The listing builds one solid part. Answer for the finished solid, in the listing's coordinates (mm). A direction names the side the tool comes from. Give positions to 0.01 mm unless a question says otherwise; leave off trailing zeros. Loops run counter-clockwise (first coordinate to the right, second up) from the corner with the lowest first, then second, coordinate; pieces in that order, holes last. Notation, with made-up numbers: (-37, 35) - (12, 35) arc R32 cw to (12, 63) - close; hole circle Ø6 at (40.25, 8). An arc over 180 degrees is marked (long way). Answer in a Markdown table with one row per item. Add a question column.
```python
from build123d import *

# Parameters (mm, degrees)
EXTRUDE_1_DEPTH     = 5
SKETCH_2_R          = 2
SKETCH_2_R_2        = 5
SKETCH_2_R_3        = 12
CUT_EXTRUDE_1_DEPTH = 96.753903315
SKETCH_3_R          = 1.5
CUT_EXTRUDE_2_DEPTH = 96.753903315
CUT_EXTRUDE_4_DEPTH = 96.753903315
FILLET_1_R          = 2
FILLET_2_R          = 2
SKETCH_5_R          = 1.5
CUT_EXTRUDE_5_DEPTH = 10


with BuildPart() as part:
    # 草图1 → 凸台-拉伸1 (new body)
    with BuildSketch(Plane(origin=(0, 0, 0), x_dir=(1, 0, 0), z_dir=(0, 1, 0))):
        Polygon((20, -34.641016151), (40, 0), (20, 34.641016151), (13.095477456, 46.6), (-83.5, 46.6), (-83.5, 26.6), (-40, 26.6), (-32.32124142, 13.3), (-40, 0), (-20, -34.641016151), align=None)
    extrude(amount=EXTRUDE_1_DEPTH)

    # 草图2 → 切除-拉伸1 (cut, through all)
    with BuildSketch(Plane(origin=(0, 5, 0), x_dir=(1, 0, 0), z_dir=(0, 1, 0))):
        with Locations(Location((0, 29, 0), (0, 0, 270))):
            Circle(SKETCH_2_R)
        with Locations(Location((25.11473671, -14.5, 0), (0, 0, 270))):
            Circle(SKETCH_2_R)
        with Locations(Location((-25.11473671, -14.5, 0), (0, 0, 270))):
            Circle(SKETCH_2_R)
        with Locations(Location((0, 19.25, 0), (0, 0, 270))):
            Circle(SKETCH_2_R_2)
        with Locations(Location((0, 0, 0), (0, 0, 270))):
            Circle(SKETCH_2_R_3)
        with Locations(Location((16.670989023, -9.625, 0), (0, 0, 270))):
            Circle(SKETCH_2_R_2)
        with Locations(Location((-16.670989023, -9.625, 0), (0, 0, 270))):
            Circle(SKETCH_2_R_2)
    extrude(amount=-CUT_EXTRUDE_1_DEPTH, mode=Mode.SUBTRACT)

    # 草图3 → 切除-拉伸2 (cut, through all)
    with BuildSketch(Plane.XZ):
        with Locations(Location((-78.5, -29.6, 0), (0, 0, 270))):
            Circle(SKETCH_3_R)
        with Locations(Location((-58.5, -29.6, 0), (0, 0, 270))):
            Circle(SKETCH_3_R)
        with Locations(Location((-58.5, -43.6, 0), (0, 0, 90))):
            Circle(SKETCH_3_R)
        with Locations(Location((-78.5, -43.6, 0), (0, 0, 90))):
            Circle(SKETCH_3_R)
    extrude(amount=-CUT_EXTRUDE_2_DEPTH, mode=Mode.SUBTRACT)

    # 草图4 → 切除-拉伸4 (cut, through all)
    with BuildSketch(Plane.XZ):
        with BuildLine():
            ThreePointArc((-16.995979196, -0.369717674), (-22.006018762, 1.167018108), (-25.550949616, 5.026489386))
            Line((-25.550949616, 5.026489386), (-28.452994616, 0))
            Line((-28.452994616, 0), (-14.226497308, -24.641016151))
            Line((-14.226497308, -24.641016151), (-8.422407308, -24.641016151))
            ThreePointArc((-8.422407308, -24.641016151), (-9.992342053, -19.641280338), (-8.818174496, -14.534090909))
            ThreePointArc((-8.818174496, -14.534090909), (-14.722431864, -8.5), (-16.995979196, -0.369717674))
        make_face()
        with BuildLine():
            Line((28.452994616, 0), (25.550949616, 5.026489386))
            ThreePointArc((25.550949616, 5.026489386), (22.006018762, 1.167018108), (16.995979196, -0.369717674))
            ThreePointArc((16.995979196, -0.369717674), (14.722431864, -8.5), (8.818174496, -14.534090909))
            ThreePointArc((8.818174496, -14.534090909), (9.700044973, -16.819130296), (10, -19.25))
            ThreePointArc((10, -19.25), (9.597501578, -22.058551844), (8.422407308, -24.641016151))
            Line((8.422407308, -24.641016151), (14.226497308, -24.641016151))
            Line((14.226497308, -24.641016151), (28.452994616, 0))
        make_face()
        with BuildLine():
            Line((17.128542308, 19.614526765), (14.226497308, 24.641016151))
            Line((14.226497308, 24.641016151), (-14.226497308, 24.641016151))
            Line((-14.226497308, 24.641016151), (-17.128542308, 19.614526765))
            ThreePointArc((-17.128542308, 19.614526765), (-12.013676709, 18.47426223), (-8.1778047, 14.903808583))
            ThreePointArc((-8.1778047, 14.903808583), (0, 17), (8.1778047, 14.903808583))
            ThreePointArc((8.1778047, 14.903808583), (12.013676709, 18.47426223), (17.128542308, 19.614526765))
        make_face()
    extrude(amount=-CUT_EXTRUDE_4_DEPTH, mode=Mode.SUBTRACT)

    # 圆角1
    fillet_1_edges = [part.edges().sort_by_distance(p)[0] for p in [
        (-8.1778047, 2.5, 14.903808583),
        (-17.128542308, 2.5, 19.614526765),
        (-14.226497308, 2.5, 24.641016151),
        (14.226497308, 2.5, 24.641016151),
        (17.128542308, 2.5, 19.614526765),
        (8.1778047, 2.5, 14.903808583),
        (16.995979196, 2.5, -0.369717674),
        (25.550949616, 2.5, 5.026489386),
        (28.452994616, 2.5, 0),
        (14.226497308, 2.5, -24.641016151),
        (8.422407308, 2.5, -24.641016151),
        (8.818174496, 2.5, -14.534090909),
        (-25.550949616, 2.5, 5.026489386),
        (-16.995979196, 2.5, -0.369717674),
        (-8.818174496, 2.5, -14.534090909),
        (-8.422407308, 2.5, -24.641016151),
        (-14.226497308, 2.5, -24.641016151),
        (-28.452994616, 2.5, 0),
    ]]
    fillet(fillet_1_edges, radius=FILLET_1_R)

    # 圆角2
    fillet_2_edges = [part.edges().sort_by_distance(p)[0] for p in [
        (-20, 2.5, 34.641016151),
        (-40, 2.5, 0),
        (-32.32124142, 2.5, -13.3),
        (-40, 2.5, -26.6),
        (-83.5, 2.5, -26.6),
        (-83.5, 2.5, -46.6),
        (13.095477456, 2.5, -46.6),
        (40, 2.5, 0),
        (20, 2.5, 34.641016151),
    ]]
    fillet(fillet_2_edges, radius=FILLET_2_R)

    # 草图5 → 切除-拉伸5 (cut)
    with BuildSketch(Plane.XZ):
        with Locations(Location((-31.401807915, -29.375609946, 0), (0, 0, 270))):
            Circle(SKETCH_5_R)
        with Locations(Location((-14.716714858, -40.403196703, 0), (0, 0, 270))):
            Circle(SKETCH_5_R)
        with Locations(Location((5.152091527, -42.690232523, 0), (0, 0, 270))):
            Circle(SKETCH_5_R)
        with Locations(Location((-34.847908473, -42.690232523, 0), (0, 0, 270))):
            Circle(SKETCH_5_R)
    extrude(amount=-CUT_EXTRUDE_5_DEPTH, mode=Mode.SUBTRACT)


solid = part.part
```
(1) Given pin 1 Ø14.5 at (x, z) = (0, 0) entering from +Y; pin 2 Ø3 at (x, y) = (-22, 3.5) entering from +Z, each flat-ended and moving along its own axis, determine where each tip first touches the part or whether it passes through.
(2) A cutting plane is placed at C-C on y = 3.25. Give the number of separate pieces and of enclosed holes in the cut face, plus the area to 3 significant figures.
(3) A cutting plane is placed at A-A on z = 6.5. Determine the outline of the cut face in (x, y).
(4) Find the intervals of material crossed by line 1 along X through (y, z) = (3.6, -43.6); line 2 along Z through (x, y) = (-12.5, 1.05); line 3 along Z through (x, y) = (-24.5, 2.6), in increasing order. Write a range as [from, to].
(5) The mould has two halves that part along Z. Classify faces 3 (the face through (-34, 2, -46.6)), 4 (the face through (-36.206, 2.465, -20.029)), 5 (the face through (0, 2, 34.641)), 6 (the face through (-9, 5, -16)): pulls with the +Z half, pulls with the -Z half, needs draft (parallel to the pull), parting line crosses it, or undercut.
(6) A tool of negligible diameter and unlimited length cuts with its end or side. For faces 1 (the face through (-21.431, 2.465, -12.162)), 2 (the face through (-83.5, 2, -37)), from which of +Z, -Z, +X, -X, +Y, -Y can it reach the whole face along a straight path? Write none if from no direction.
(7) A cutting plane is placed at B-B on x = -68. Determine the outline of the cut face in (y, z), plus the area to 3 significant figures.
Evaluation:
| question | item | result |
|---|---|---|
| 1 | pin 1 | passes through |
| 1 | pin 2 | stops at z = 33.76 |
| 2 | separate pieces | 1 |
| 2 | enclosed holes | 18 |
| 2 | area | 4,470 mm² |
| 3 | outline | (-36.25, 0) - (-20.57, 0) - (-20.57, 5) - (-36.25, 5) - close; (-12.77, 0) - (-10.09, 0) - (-10.09, 5) - (-12.77, 5) - close; (10.09, 0) - (12.77, 0) - (12.77, 5) - (10.09, 5) - close; (20.57, 0) - (36.25, 0) - (36.25, 5) - (20.57, 5) - close |
| 4 | line 1 | x = [-83.5, -80], [-77, -60], [-57, -36.04], [-33.66, 3.96], [6.34, 14.83] |
| 4 | line 2 | z = [-46.6, -24.64], [-11.52, 6.87], [12.38, 18.71], [24.64, 34.64] |
| 4 | line 3 | z = [-46.6, -6.85], [3.16, 12.6], [16.4, 26.85] |
| 5 | face 3 | pulls with the -Z half |
| 5 | face 4 | undercut |
| 5 | face 5 | pulls with the +Z half |
| 5 | face 6 | needs draft |
| 6 | face 1 | +Y, -Y |
| 6 | face 2 | +Z, -Z, -X, +Y, -Y |
| 7 | outline | (0, -46.6) - (5, -46.6) - (5, -26.6) - (0, -26.6) - close |
| 7 | area | 100 mm² |
